Here's how the part is built. I have some questions about the finished solid (model axes, mm). A direction names the side the tool comes from. Round coordinates to 2 decimals unless told otherwise and drop trailing zeros. Loops run counter-clockwise (first coordinate to the right, second up) from the corner with the lowest first, then second, coordinate; pieces in that order, holes last. Notation, with made-up numbers: (-38.75, 51) - (-19.75, 51) arc R21 cw to (-19.75, 56) - close; hole circle Ø11 at (52.25, 15). An arc over 180 degrees is marked (long way). Answer as a JSON object with one key per item and string values. Group by question number.
1) If I drill on line 1 along Y through (x, z) = (-5.9, 48.5) (3 decimals); line 2 along X through (y, z) = (-12, 79); line 3 along Y through (x, z) = (1, 16), over which ranges is the centre line in solid material (lowest first)? Write a range as [from, to].
2) If we mould it in two halves opening along Z, with no side actions, what happens to faces 6 (the face through (-5.879, 39.06, 49.874)), 7 (the face through (-6, 1, 101)), 8 (the face through (-6, 24, 45))? For each: pulls with the +Z half, pulls with the -Z half, needs draft (parallel to the pull), parting line crosses it, or undercut.
3) I want a section at B-B, the plane y = -4. Please give me the cut outline in (x, z), then the cut area to 3 significant figures.
4) I want a section at D-D, the plane x = 4. Please give me the cut outline in (y, z), then the cut area to 3 significant figures.
5) I want a section at C-C, the plane z = 29. Please give me the cut outline in (x, y), then the cut area to 3 significant figures.
6) I want a section at A-A, the plane y = -19. Please give me the cut outline in (x, z) (3 decimals), then the cut area to 4 significant figures.
7) Which directions (+Z, -Z, +X, -X, +Y, -Y) give clear straight access to the entire face, cutting with the end or side of a thin tool? Please do faces 1 (the face through (-6, -23, 45)), 2 (the face through (-6, -42.5, 73)), 3 (the face through (0, 7.4, 17)), 4 (the face through (-5.88, -41.64, 100.1)), 5 (the face through (1, 0, 35)).
8) Will these pins go through, and if not, where does the flat tip stop? P1, Ø3, axis at y = 39, z = 97.5, coming from the -X side; P2, Ø4.5, axis at x = -1.5, z = 22.5, coming from the -Y side; P3, Ø4.5, axis at y = -19, z = 97.5, coming from the +X side; P4, Ø3.5, axis at x = -6, y = -16, coming from the -Z side.
from build123d import *

# Parameters (mm, degrees)
SKETCH1_W           = 14.8
SKETCH1_H           = 14.8
BOSS_EXTRUDE1_DEPTH = 35
SKETCH3_W           = 3
SKETCH3_H           = 14.8
BOSS_EXTRUDE3_DEPTH = 10
SKETCH5_W           = 3
SKETCH5_H           = 85
BOSS_EXTRUDE4_DEPTH = 56
SKETCH6_R           = 1.375
CUT_EXTRUDE1_DEPTH  = 5
FILLET2_R           = 3


with BuildPart() as part:
    # Sketch1 → Boss-Extrude1 (new body)
    with BuildSketch(Plane.XY):
        Rectangle(SKETCH1_W, SKETCH1_H)
    extrude(amount=BOSS_EXTRUDE1_DEPTH)

    # Sketch3 → Boss-Extrude3 (add)
    with BuildSketch(Plane.XY.offset(35)):
        with Locations((-5.9, 0)):
            Rectangle(SKETCH3_W, SKETCH3_H)
    extrude(amount=BOSS_EXTRUDE3_DEPTH)

    # Sketch5 → Boss-Extrude4 (add)
    with BuildSketch(Plane.XY.offset(45)):
        with Locations((-5.9, 0)):
            Rectangle(SKETCH5_W, SKETCH5_H)
    extrude(amount=BOSS_EXTRUDE4_DEPTH)

    # Sketch6 → Cut-Extrude1 (cut)
    with BuildSketch(Plane(origin=(-4.4, 0, 0), x_dir=(0, 0, -1), z_dir=(1, 0, 0))):
        with Locations((-97.5, 39)):
            Circle(SKETCH6_R)
        with Locations((-48.5, 39)):
            Circle(SKETCH6_R)
        with Locations((-48.5, -19)):
            Circle(SKETCH6_R)
        with Locations((-97.5, -19)):
            Circle(SKETCH6_R)
    extrude(amount=-CUT_EXTRUDE1_DEPTH, mode=Mode.SUBTRACT)

    # Fillet2
    fillet2_edges = [part.edges().sort_by_distance(p)[0] for p in [
        (-5.9, -42.5, 45),
        (-5.9, 42.5, 45),
        (-5.9, -42.5, 101),
        (-5.9, 42.5, 101),
    ]]
    fillet(fillet2_edges, radius=FILLET2_R)


solid = part.part
Outcome:
{
 "1": {"line 1": "[-42.5, -20.375], [-17.625, 37.625], [40.375, 42.5]", "line 2": "[-7.4, -4.4]", "line 3": "[-7.4, 7.4]"},
 "2": {"face 6": "undercut", "face 7": "pulls with the +Z half", "face 8": "pulls with the -Z half"},
 "3": {"outline": "(-7.4, 0) - (7.4, 0) - (7.4, 35) - (-4.4, 35) - (-4.4, 101) - (-7.4, 101) - close", "area": "716 mm^2"},
 "4": {"outline": "(-7.4, 0) - (7.4, 0) - (7.4, 35) - (-7.4, 35) - close", "area": "518 mm^2"},
 "5": {"outline": "(-7.4, -7.4) - (7.4, -7.4) - (7.4, 7.4) - (-7.4, 7.4) - close", "area": "219 mm^2"},
 "6": {"outline": "(-7.4, 45) - (-4.4, 45) - (-4.4, 47.125) - (-7.4, 47.125) - close; (-7.4, 49.875) - (-4.4, 49.875) - (-4.4, 96.125) - (-7.4, 96.125) - close; (-7.4, 98.875) - (-4.4, 98.875) - (-4.4, 101) - (-7.4, 101) - close", "area": "151.5 mm^2"},
 "7": {"face 1": "-Z, +X, -X, -Y", "face 2": "+Z, -Z, +X, -X, -Y", "face 3": "-Z, +X, -X, +Y", "face 4": "+Z, +X, -X, -Y", "face 5": "+Z, +X, +Y, -Y"},
 "8": {"P1": "x = -7.4", "P2": "y = -7.4", "P3": "x = -4.4", "P4": "z = 45"}
}
